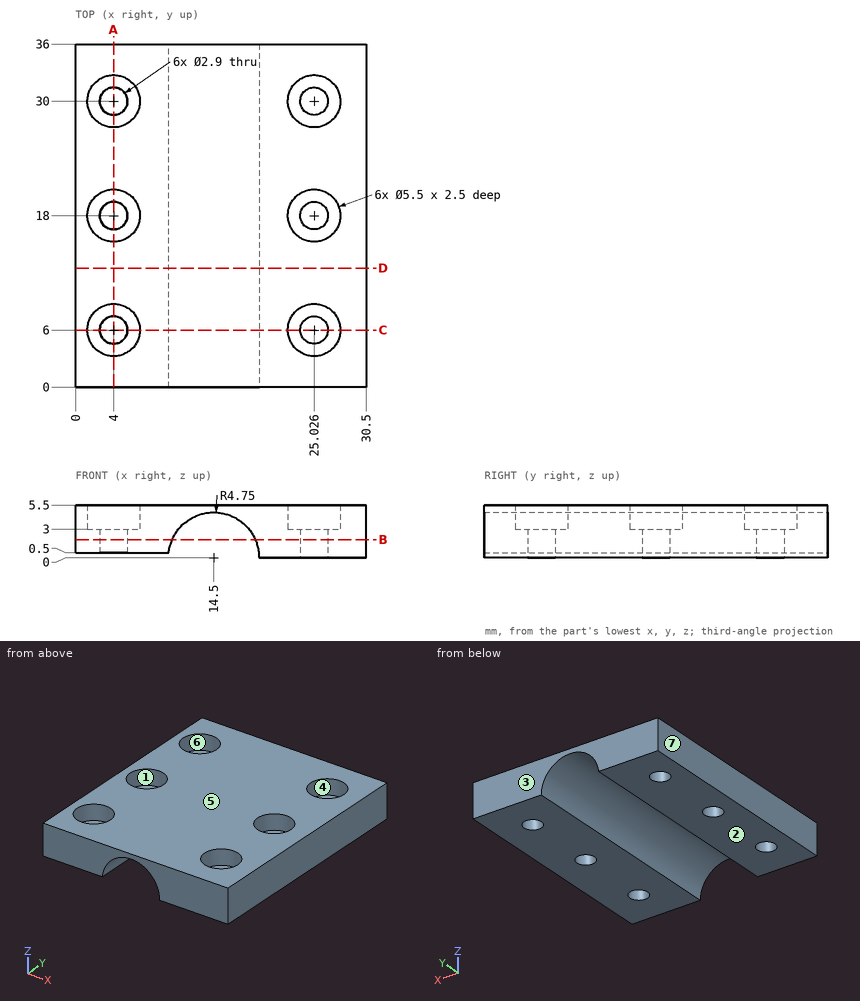
For this review, use the dimensioned drawing (mm, ordinates from the lowest corner) and the shaded views. A direction names the side the tool comes from. Round coordinates to 2 decimals unless told otherwise and drop trailing zeros. Order: outer loops, then holes, each group sorted by start corner. A loop starts at its lowest first (then second) coordinate and runs counter-clockwise, first axis right, second up. Notation, with made-up numbers: M -5,23.5 L 15,23.5 A20 ccw 15,51.5 Z; hole C 40.25,80 d2. An arc over 180 degrees is marked long. Use a Markdown table: item, result.
1) Insertion check: pin 1 (5 mm diameter, centred on x = 25.03, y = 6, fed in from +Z); pin 2 (11 mm diameter, centred on x = 4.5, y = 19.5, fed in from -Z); pin 3 (2.5 mm diameter, centred on x = 25.03, y = 18, fed in from -Z). Each pin has a flat end and moves straight along its axis. Give the tip position at first contact, or say it passes through.
Report:
| item | result |
|---|---|
| pin 1 | z = 3 |
| pin 2 | z = 0.5 |
| pin 3 | through |
2) Tool access review of the marked faces 1, 2 and 3: name each direction out of +Z, -Z, +X, -X, +Y, -Y from which nothing blocks a thin tool from reaching the whole face with its end or side.
Report:
| item | result |
|---|---|
| face 1 | +Z |
| face 2 | -Z, -X, +Y, -Y |
| face 3 | +Z, -Z, +X, -X, +Y |
3) Consider section A-A (x = 4). Write out the cut boundary in (y, z).
Report:
| item | result |
|---|---|
| outline | M 0,0.5 L 4.55,0.5 L 4.55,3 L 3.25,3 L 3.25,5.5 L 0,5.5 Z; M 7.45,0.5 L 16.55,0.5 L 16.55,3 L 15.25,3 L 15.25,5.5 L 8.75,5.5 L 8.75,3 L 7.45,3 Z; M 19.45,0.5 L 28.55,0.5 L 28.55,3 L 27.25,3 L 27.25,5.5 L 20.75,5.5 L 20.75,3 L 19.45,3 Z; M 31.45,0.5 L 36,0.5 L 36,5.5 L 32.75,5.5 L 32.75,3 L 31.45,3 Z |
4) Consider section D-D (y = 12.5). Write out the cut boundary in (x, z), then the cut area to 3 significant figures.
Report:
| item | result |
|---|---|
| outline | M 0,0.5 L 9.78,0.5 A4.75 cw 19.25,0 L 30.5,0 L 30.5,5.5 L 0,5.5 Z |
| area | 127 mm^2 |
5) Draft analysis for pull direction X (two halves, no side actions). For the marked faces 4, 5, 6 and 7, state which applies: released by +X, released by -X, zero draft, split by the parting line, or undercut.
Report:
| item | result |
|---|---|
| face 4 | undercut |
| face 5 | zero draft |
| face 6 | undercut |
| face 7 | released by -X |
6) Consider section B-B (z = 1.9). Write out the cut boundary in (x, y).
Report:
| item | result |
|---|---|
| outline | M 0,0 L 10.15,0 L 10.15,36 L 0,36 Z; M 18.85,0 L 30.5,0 L 30.5,36 L 18.85,36 Z; hole C 4,6 d2.9; hole C 4,18 d2.9; hole C 4,30 d2.9; hole C 25.03,6 d2.9; hole C 25.03,18 d2.9; hole C 25.03,30 d2.9 |
7) Consider section C-C (y = 6). Write out the cut boundary in (x, z).
Report:
| item | result |
|---|---|
| outline | M 0,0.5 L 2.55,0.5 L 2.55,3 L 1.25,3 L 1.25,5.5 L 0,5.5 Z; M 5.45,0.5 L 9.78,0.5 A4.75 cw 19.25,0 L 23.58,0 L 23.58,3 L 22.28,3 L 22.28,5.5 L 6.75,5.5 L 6.75,3 L 5.45,3 Z; M 26.48,0 L 30.5,0 L 30.5,5.5 L 27.78,5.5 L 27.78,3 L 26.48,3 Z |
8) Wall thickness on line 1 along Y through (x, z) = (4, 1.25); line 2 along Y through (x, z) = (24.5, 5.1); line 3 along X through (y, z) = (30, 1): over which ranges is each line inside the solid? List them lowest first. Write a range as [from, to].
Report:
| item | result |
|---|---|
| line 1 | [0, 4.55], [7.45, 16.55], [19.45, 28.55], [31.45, 36] |
| line 2 | [0, 3.3], [8.7, 15.3], [20.7, 27.3], [32.7, 36] |
| line 3 | [0, 2.55], [5.45, 9.86], [19.14, 23.58], [26.48, 30.5] |
